Autodesk Inventor part; units mm, degrees
ref_plane "YZ Plane" through (0, 0, 0) normal (1, 0, 0) x (0, 1, 0)
ref_plane "XZ Plane" through (0, 0, 0) normal (0, 1, 0) x (-1, 0, 0)
ref_plane "XY Plane" through (0, 0, 0) normal (0, 0, 1) x (1, 0, 0)
sketch "Sketch1" plane through (0, 0, 0) normal (0, 0, 1) x (1, 0, 0)
  arc A0 (5.5, 7) -> (3.5, 9) centre (3.5, 7) ccw
  line L0 (3.5, 9) -> (-5.5, 9)
  line L1 (-5.5, -9) -> (-5.5, 9)
  line L2 (-5.5, -9) -> (3.5, -9)
  arc A1 (3.5, -9) -> (5.5, -7) centre (3.5, -7) ccw
  line L3 (5.5, -7) -> (5.5, 7)
  circle A2 centre (0, 4) radius 2.25 construction
  circle A3 centre (0, -4) radius 2.25 construction
  arc A4 (5.5, 39) -> (3.5, 41) centre (3.5, 39) ccw
  line L4 (3.5, 41) -> (-5.5, 41)
  line L5 (-5.5, 23) -> (-5.5, 41)
  line L6 (-5.5, 23) -> (3.5, 23)
  arc A5 (3.5, 23) -> (5.5, 25) centre (3.5, 25) ccw
  line L7 (5.5, 25) -> (5.5, 39)
  circle A6 centre (0, 36) radius 2.25 construction
  circle A7 centre (0, 28) radius 2.25 construction
  circle A8 centre (0, 4) radius 1.75
  circle A9 centre (0, -4) radius 1.75
  circle A10 centre (0, 28) radius 1.75
  circle A11 centre (0, 36) radius 1.75
  line L8 (6.4713, 13.5) -> (-5.5, 13.5) construction
  line L9 (-5.5, 18.5) -> (6.4713, 18.5) construction
  line L10 (6.5, -9) -> (9.6, -9)
  line L11 (9.6, -9) -> (9.6, 41)
  line L12 (9.6, 41) -> (6.5, 41)
  line L13 (6.5, 41) -> (6.5, -9)
  line L14 (-1, 9) -> (-1, 23) construction
  line L15 (-1, 16) -> (6.5, 16) construction
  line L16 (3.5, -12) -> (12.6, -12)
  line L17 (12.6, -12) -> (12.6, 44)
  line L18 (12.6, 44) -> (3.5, 44)
  line L19 (3.5, 44) -> (3.5, -12)
  point P0 (0, 0)
  dimension "d0" = 3.5
  dimension "d1" = 3.5
  dimension "d2" = 3.5
  dimension "d3" = 3.5
  dimension "d4" = 3.1
  dimension "d5" = 50
  dimension "d7" = 3
extrude "Extrusion1" add sketch "Sketch1" along normal blind 5
sketch "Sketch2" plane through (0, 0, 5) normal (0, 0, 1) x (1, 0, 0)
  line L0 (12.6, 44) -> (3.5, 44)
  line L1 (3.5, -12) -> (12.6, -12)
  line L2 (12.6, -12) -> (12.6, 44)
  line L3 (12.6, -12) -> (3.5, -12)
  line L4 (3.5, -12) -> (3.5, 44)
  line L5 (3.5, 44) -> (12.6, 44)
  line L6 (12.6, 44) -> (12.6, -12)
  line L7 (6.5, -9) -> (6.5, 41)
  line L8 (9.6, -9) -> (6.5, -9)
  line L9 (6.5, 41) -> (9.6, 41)
  line L10 (9.6, 41) -> (9.6, -9)
  line L11 (9.6, -9) -> (6.5, -9)
  line L12 (6.5, -9) -> (6.5, 41)
  point P0 (0, 0)
extrude "Extrusion2" add sketch "Sketch2" along normal blind 5
sketch "Sketch3" plane through (12.6, -12, 0) normal (1, 0, 0) x (0, 0, -1)
  circle A0 centre (-18, 40) radius 1.75
  arc A1 (-18.5567, 43.9611) -> (-18.5567, 36.0389) centre (-18, 40) ccw
  line L0 (-18.5567, 36.0389) -> (-10, 34.8364)
  line L1 (-10, 0) -> (-10, 56)
  line L2 (-18.5567, 43.9611) -> (-10, 45.1636)
  line L3 (-18, 40) -> (-10, 40) construction
  line L4 (-33.1913, 28) -> (0, 28)
  line L5 (0, 0) -> (0, 56)
  circle A2 centre (-18, 16) radius 1.75
  arc A3 (-18.5567, 19.9611) -> (-18.5567, 12.0389) centre (-18, 16) ccw
  line L6 (-18.5567, 19.9611) -> (-10, 21.1636)
  line L7 (-18.5567, 12.0389) -> (-10, 10.8364)
  line L8 (-18, 16) -> (-10, 16) construction
  point P0 (0, 12)
  point P1 (-14, 40)
  point P2 (-10, 28)
  point P3 (-10, 28)
  point P4 (-14, 16)
  dimension "d12" = 3.5
  dimension "d13" = 8
  dimension "d14" = 8
  dimension "d15" = 4
  dimension "d16" = 8
  dimension "d17" = 12
extrude "Extrusion3" add sketch "Sketch3" against normal up to surface (3 mm away)
sketch "Sketch4" plane through (0, 0, 5) normal (0, 0, 1) x (1, 0, 0)
  point P0 (0, 0)
chamfer "Chamfer1" distance 3 angle 45 2 edges at (8.05, 44, 0) (8.05, -12, 0)
properties part number "Lysekrone_adapter"
Read the model definition and answer for the solid it produces. Units are mm, in the model's axes. A direction names the side the tool comes from. Round coordinates to 2 decimals unless told otherwise and drop trailing zeros. Loops run counter-clockwise (first coordinate to the right, second up) from the corner with the lowest first, then second, coordinate; pieces in that order, holes last.
Q1. Section B-B on y = 4 is taken. Write down the section's boundary in (x, z), and give its area (3 significant figures).
Q2. Section D-D on x = 0 is taken. Write down the section's boundary in (y, z), and give its area (3 significant figures).
Q3. Section C-C on y = 18.5 is taken. Write down the section's boundary in (x, z).
Q4. Which of the six approach directions +Z, -Z, +X, -X, +Y, -Y give full straight-line access (tool end or side, diameter ignored) to faces 1 (the face through (11.121, 23.446, 14.338)), 2 (the face through (-1, 0, 5)), 3 (the face through (9.6, 16, 6))?
Q5. Consider probe 1 along Y at (x, z) = (0, 2.65); probe 2 along X at (y, z) = (7.5, 6.5); probe 3 along X at (y, z) = (39, 4.25). Determine where each line is inside the solid, lowest interval first.
Q6. Section A-A on x = -2.75 is taken. Write down the section's boundary in (y, z).
Q7. Determine the mould class of faces 4 (the face through (-1, 23, 2)), 5 (the face through (-5.5, 0, 2)), 6 (the face through (8, 44, 6)), 7 (the face through (-0.38, 5.71, 2.46)) for opening direction Y: released by +Y, released by -Y, zero draft, split by the parting line, or undercut.
Q8. Each of these flat-tipped pins is pushed along its axis until it touches: pin 1 (2.5 mm diameter, centred on x = 8, y = 11.5, fed in from +Z); pin 2 (1.5 mm diameter, centred on x = 11, y = 13.5, fed in from +Z); pin 3 (2.5 mm diameter, centred on x = 0, y = 2, fed in from +Z); pin 4 (5.5 mm diameter, centred on x = 0.5, z = 2.5, fed in from -Y). Where does it stop, or does it pass through?
Output:
1. outline: (-5.5, 0) - (-1.75, 0) - (-1.75, 5) - (-5.5, 5) - close; (1.75, 0) - (6.5, 0) - (6.5, 10) - (3.5, 10) - (3.5, 5) - (1.75, 5) - close; (9.6, 0) - (12.6, 0) - (12.6, 16.25) - (9.6, 16.25) - close; (9.6, 19.75) - (12.6, 19.75) - (12.6, 22) - (9.6, 22) - close
1. area: 113 mm2
2. outline: (-9, 0) - (-5.75, 0) - (-5.75, 5) - (-9, 5) - close; (-2.25, 0) - (2.25, 0) - (2.25, 5) - (-2.25, 5) - close; (5.75, 0) - (9, 0) - (9, 5) - (5.75, 5) - close; (23, 0) - (26.25, 0) - (26.25, 5) - (23, 5) - close; (29.75, 0) - (34.25, 0) - (34.25, 5) - (29.75, 5) - close; (37.75, 0) - (41, 0) - (41, 5) - (37.75, 5) - close
2. area: 110 mm2
3. outline: (3.5, 0) - (6.5, 0) - (6.5, 10) - (3.5, 10) - close; (9.6, 0) - (12.6, 0) - (12.6, 10) - (9.6, 10) - close
4. face 1: +Z, +X, -X
4. face 2: +Z, -X, +Y, -Y
4. face 3: +Z, -Z
5. probe 1: y = -9 to -5.75, -2.25 to 2.25, 5.75 to 9, 23 to 26.25, 29.75 to 34.25, 37.75 to 41
5. probe 2: x = 3.5 to 6.5, 9.6 to 12.6
5. probe 3: x = -5.5 to 6.5, 9.6 to 12.6
6. outline: (-9, 0) - (9, 0) - (9, 5) - (-9, 5) - close; (23, 0) - (41, 0) - (41, 5) - (23, 5) - close
7. face 4: undercut
7. face 5: zero draft
7. face 6: released by +Y
7. face 7: undercut
8. pin 1: passes through
8. pin 2: stops at z = 10
8. pin 3: stops at z = 5
8. pin 4: stops at y = -9
